Autodesk Fusion 360 part; units mm, degrees
sketch "Sketch1" plane through (0, 0, 0) normal (0, 0, 1) x (1, 0, 0)
  circle A0 centre (0, 0) radius 25
  circle A1 centre (0, 0) radius 30
  circle A2 centre (0, 0) radius 33
  dimension "d1" = 50
  dimension "d2" = 60
  dimension "d3" = 66
extrude "Extrude1" add sketch "Sketch1" along normal blind 3 contours A1 | A2
sketch "Sketch2" plane through (0, 0, 3) normal (0, 0, 1) x (-1, 0, 0)
  circle A0 centre (0, 0) radius 25
  circle A1 centre (0, 0) radius 33
  circle A2 centre (0, 0) radius 30
  circle A3 centre (0, 0) radius 33
extrude "Extrude2" add sketch "Sketch2" along normal blind 15 contours A1 A3
fillet "Fillet1" radius 1 2 edges at (27.9698, -10.8485, 18) (30.7668, 11.9333, 18)
fillet "Fillet2" radius 1 1 edges at (-30.7668, -11.9333, 0)
move_face "OffsetFaces1" offset -0.2 1 faces at (-29.8509, 2.987, 7.6667)
Work out the finished part from the listing and answer in its coordinate system (mm). A direction names the side the tool comes from. Give positions to 0.01 mm unless a question says otherwise; leave off trailing zeros. Loops run counter-clockwise (first coordinate to the right, second up) from the corner with the lowest first, then second, coordinate; pieces in that order, holes last. Notation, with made-up numbers: M 75,84.25 L 103,84.25 A10 ccw 103,97.25 Z; hole C -18.5,12.25 d3. An arc over 180 degrees is marked long. One line per item, written item: value. Start each with the question number.
1. Determine the mould class of faces 1 (the face through (6.55, -29.48, 9.9)), 2 (the face through (12, -29, 17.8)), 3 (the face through (-2.16, 32.73, 8.89)) for opening direction Y: released by +Y, released by -Y, zero draft, split by the parting line, or undercut.
2. Find the intervals of material crossed by probe 1 along Y at (x, z) = (0, 2.1); probe 2 along X at (y, z) = (0, 8), in increasing order.
3. Find section B-B (z = 6). Give the vertices of the cut face in (x, y), and give its area (3 significant figures).
4. Each of these flat-tipped pins is pushed along its axis until it touches: P1, Ø1.5, axis at y = 11.5, z = 5, coming from the -X side; P2, Ø6, axis at x = -24.5, z = 8, coming from the +Y side. Where does it stop, or does it pass through?
5. Which of the six approach directions +Z, -Z, +X, -X, +Y, -Y give full straight-line access (tool end or side, diameter ignored) to faces 4 (the face through (23.846, -7.509, 1.58)), 5 (the face through (-11, 23, 3))?
Reported:
1. face 1: undercut
1. face 2: zero draft
1. face 3: split by the parting line
2. probe 1: y = -32.8 to -25, 25 to 32.8
2. probe 2: x = -32.8 to -30.2, 30.2 to 32.8
3. outline: C 0,0 d65.6; hole C 0,0 d60.4
3. area: 515 mm²
4. P1: stops at x = -30.99
4. P2: stops at y = 24.77
5. face 4: +Z, -Z
5. face 5: +Z
